from build123d import *

# Parameters (mm, degrees)
SKETCH1_R                = 2.8
SKETCH1_R_2              = 2.25
BOSS_EXTRUDE1_DEPTH      = 5
SKETCH3_W                = 60
SKETCH3_H                = 10
BOSS_EXTRUDE3_DEPTH      = 27.5
SKETCH4_R                = 2.5
CUT_EXTRUDE1_DEPTH       = 61.993852149
CHAMFER1_SIZE            = 0.75
BOSS_EXTRUDE4_DEPTH      = 30
BOSS_EXTRUDE4_DEPTH_BACK = 40
SKETCH5_W                = 10
SKETCH5_H                = 3
CHAMFER2_SIZE            = 10
CHAMFER3_SIZE            = 5
SKETCH7_W                = 2
SKETCH7_H                = 30
CUT_EXTRUDE2_DEPTH       = 83.462112512
BOSS_EXTRUDE5_DEPTH      = 5
CUT_EXTRUDE3_DEPTH       = 79.89866919
SKETCH10_R               = 2.5
CUT_EXTRUDE4_DEPTH       = 2


with BuildPart() as part:
    # Sketch1 → Boss-Extrude1 (new body)
    with BuildSketch(Plane(origin=(0, 0, 0), x_dir=(1, 0, 0), z_dir=(0, 1, 0))):
        Polygon((-30, 0), (-30, 40), (30, 40), (30, 0), (30, -2), (-30, -2), align=None)
        with Locations(Location((-12.5, 22.5, 0), (0, 0, 270))):
            Circle(SKETCH1_R, mode=Mode.SUBTRACT)
        with Locations(Location((12.5, 22.5, 0), (0, 0, 270))):
            Circle(SKETCH1_R, mode=Mode.SUBTRACT)
        with Locations(Location((-17.5, 15, 0), (0, 0, 270))):
            Circle(SKETCH1_R_2, mode=Mode.SUBTRACT)
        with Locations(Location((17.5, 15, 0), (0, 0, 270))):
            Circle(SKETCH1_R_2, mode=Mode.SUBTRACT)
        with Locations(Location((0, 6, 0), (0, 0, 270))):
            Circle(SKETCH1_R, mode=Mode.SUBTRACT)
    extrude(amount=BOSS_EXTRUDE1_DEPTH)

    # Sketch3 → Boss-Extrude3 (add)
    with BuildSketch(Plane(origin=(0, 5, 0), x_dir=(1, 0, 0), z_dir=(0, 1, 0))):
        with Locations((0, 35)):
            Rectangle(SKETCH3_W, SKETCH3_H)
    extrude(amount=BOSS_EXTRUDE3_DEPTH)

    # Sketch4 → Cut-Extrude1 (cut, through all)
    with BuildSketch(Plane(origin=(0, 0, -40), x_dir=(-1, 0, 0), z_dir=(0, 0, -1))):
        with Locations((-17.8, 25)):
            Circle(SKETCH4_R)
        with Locations((17.8, 25)):
            Circle(SKETCH4_R)
    extrude(amount=-CUT_EXTRUDE1_DEPTH, mode=Mode.SUBTRACT)

    # Chamfer1
    chamfer1_edges = [part.edges().sort_by_distance(p)[0] for p in [
        (-12.5, 5, -25.3),
        (12.5, 5, -25.3),
        (0, 5, -8.8),
    ]]
    chamfer(chamfer1_edges, length=CHAMFER1_SIZE)

    # Sketch5 → Boss-Extrude4 (add, two sides: drawn at the far end of the back side and taken through both)
    with BuildSketch(Plane.XZ.offset(-BOSS_EXTRUDE4_DEPTH_BACK)):
        Polygon((18, 13), (15, 10), (15, 2), (30, 2), (30, 13), align=None)
        with Locations((22.5, 8)):
            Rectangle(SKETCH5_W, SKETCH5_H, mode=Mode.SUBTRACT)
    extrude(amount=BOSS_EXTRUDE4_DEPTH + BOSS_EXTRUDE4_DEPTH_BACK)

    # Chamfer2
    chamfer2_edges = [part.edges().sort_by_distance(p)[0] for p in [
        (22.5, 5, 2),
    ]]
    chamfer(chamfer2_edges, length=CHAMFER2_SIZE)

    # Chamfer3
    chamfer3_edges = [part.edges().sort_by_distance(p)[0] for p in [
        (15, 2.5, 2),
        (15, 5, -3),
    ]]
    chamfer(chamfer3_edges, length=CHAMFER3_SIZE)

    # Sketch7 → Cut-Extrude2 (cut, through all)
    with BuildSketch(Plane(origin=(30, 0, 0), x_dir=(0, 0, -1), z_dir=(1, 0, 0))):
        with Locations((-3, -15)):
            Rectangle(SKETCH7_W, SKETCH7_H)
    extrude(amount=-CUT_EXTRUDE2_DEPTH, mode=Mode.SUBTRACT)

    # Sketch8 → Boss-Extrude5 (add)
    with BuildSketch(Plane(origin=(30, 0, 0), x_dir=(0, 0, -1), z_dir=(1, 0, 0))):
        Polygon((30, 32.5), (-2, 32.5), (-2, 15), (8, 5), (30, 5), align=None)
    extrude(amount=-BOSS_EXTRUDE5_DEPTH)

    # Sketch9 → Cut-Extrude3 (cut, through all)
    with BuildSketch(Plane.ZY.offset(-25)):
        Polygon((-30, 32.5), (-30, 5), (-8, 5), (2, 15), (2, 32.5), align=None)
    extrude(amount=-CUT_EXTRUDE3_DEPTH, mode=Mode.SUBTRACT)

    # Sketch10 → Cut-Extrude4 (cut)
    with BuildSketch(Plane(origin=(0, 0, -40), x_dir=(-1, 0, 0), z_dir=(0, 0, -1))):
        with Locations((0, 25)):
            Circle(SKETCH10_R)
    extrude(amount=-CUT_EXTRUDE4_DEPTH, mode=Mode.SUBTRACT)


solid = part.part
Input: part model. Units: mm. Frame: model coordinates. A direction names the side the tool comes from. Round coordinates to 2 decimals unless told otherwise and drop trailing zeros. Write each loop counter-clockwise with the first axis right and the second up, starting at its lowest first coordinate (ties: lowest second). Pieces come first, ordered by that corner, then holes.
1) Cut plane B-B (x = 12.5). Return the cut outline in (y, z), then the cut area to 3 significant figures.
2) Reachability of faces 1 (the flat face through (0, 25, -38)), 2 (the flat face through (-10, 2, 2)), 3 (the flat face through (0, 32.5, -35)), 4 (the flat face through (27.5, 5, 8)) from +Z, -Z, +X, -X, +Y, -Y: full face, straight path, thin tool, end or side. Return the list, or none.
3) Cut plane D-D (z = -6). Return the cut outline in (x, y), then the cut area to 3 significant figures.
4) Ray query, L1, parallel to X at y = 3.2, z = -15; L2, parallel to X at y = 6, z = 10; L3, parallel to Y at x = 17.8, z = -38. Return the intervals inside material, ascending.
5) Cut plane A-A (y = 19.5). Return the cut outline in (x, z), then the cut area to 4 significant figures.
6) Contact query for flat-ended pins moving along their axis: P1, Ø7.5, axis at x = 12.5, z = -22.5, coming from the -Y side; P2, Ø5, axis at x = 1.5, y = 9, coming from the +Z side; P3, Ø12, axis at x = -6.5, z = -29, coming from the +Y side; P4, Ø5, axis at x = -12.5, z = -22.5, coming from the +Y side. Output: stop coordinate, or through.
7) Cut plane C-C (z = -15). Return the cut outline in (x, y), then the cut area to 3 significant figures.
8) Draft query along Z for faces 5 (the cylindrical face through (-17.47, 27.48, -35.07)), 6 (the flat face through (0, 19, -30)), 7 (the flat face through (22, 10, -3)), 8 (the flat face through (0, 16, -40)). Return one class per face: pulls with the +Z half, pulls with the -Z half, needs draft (parallel to the pull), parting line crosses it, or undercut.
Geometry says:
1. outline: (0, -40) - (32.5, -40) - (32.5, -30) - (5, -30) - (5, -26.05) - (4.25, -25.3) - (0, -25.3) - close; (0, -19.7) - (4.25, -19.7) - (5, -18.95) - (5, -8) - (7.5, -5.5) - (7.5, 4.5) - (0, 4.5) - close
1. area: 497 mm2
2. face 1: -Z
2. face 2: +Z, -X, +Y, -Y
2. face 3: -Z, +X, -X, +Y
2. face 4: +Y, -Y
3. outline: (-30, 0) - (-2.8, 0) - (-2.8, 4.25) - (-3.55, 5) - (-30, 5) - close; (2.8, 0) - (30, 0) - (30, 7) - (12, 7) - (10, 5) - (3.55, 5) - (2.8, 4.25) - close
3. area: 309 mm2
4. L1: x = -30 to -19.75, -15.25 to 15.25, 19.75 to 30
4. L2: x = 15 to 30
4. L3: y = 0 to 22.5, 27.5 to 32.5
5. outline: (-30, -40) - (30, -40) - (30, -30) - (-30, -30) - close; (15, 2) - (30, 2) - (30, 13) - (18, 13) - (15, 10) - close; hole (17.5, 6.5) - (27.5, 6.5) - (27.5, 9.5) - (17.5, 9.5) - close
5. area: 730.5 mm2
6. P1: stops at y = 0
6. P2: stops at z = -30
6. P3: stops at y = 32.5
6. P4: passes through
7. outline: (-30, 0) - (-19.75, 0) - (-19.75, 5) - (-30, 5) - close; (-15.25, 0) - (15.25, 0) - (15.25, 5) - (-15.25, 5) - close; (19.75, 0) - (30, 0) - (30, 5) - (19.75, 5) - close
7. area: 255 mm2
8. face 5: needs draft
8. face 6: undercut
8. face 7: undercut
8. face 8: pulls with the -Z half
